Geometry check sheet. Reference: the model listing, model coordinates, mm. Give positions to 0.01 mm unless a question says otherwise; leave off trailing zeros. Order: outer loops, then holes, each group sorted by start corner. A loop starts at its lowest first (then second) coordinate and runs counter-clockwise, first axis right, second up. Notation, with made-up numbers: M 21,18 L 39,18 A10 ccw 39,27 Z; hole C 5,64 d2. An arc over 180 degrees is marked long. Answer as CSV lines item,"result". Start each with the question number.
Q1. Go/stop test with flat-tipped pins: pin 1 (2 mm diameter, centred on x = 30, y = 1.5, fed in from -Z); pin 2 (1 mm diameter, centred on y = 1, z = 15, fed in from -X); pin 3 (0.8 mm diameter, centred on x = -2, y = -1.5, fed in from +Z). Record where each tip stops, or that it passes through.
Q2. Thickness scan on line 1 (X direction, y = -1.5, z = 22); line 2 (Z direction, x = -13, y = 0.25). Record the ranges inside material, lowest first.
Q3. Section check A-A, the plane y = -1.1. Record the boundary of the cut face in (x, z).
```python
from build123d import *

# Parameters (mm, degrees)
BOSS_EXTRUDE1_DEPTH = 2.54
BOSS_EXTRUDE2_DEPTH = 2.54
FILLET1_R           = 2.54


with BuildPart() as part:
    # Sketch1 → Boss-Extrude1 (new body)
    with BuildSketch(Plane(origin=(0, 0, 0), x_dir=(1, 0, 0), z_dir=(0, 1, 0))):
        with BuildLine():
            Line((-44.45, 50.8), (44.45, 50.8))
            ThreePointArc((44.45, 50.8), (48.940128061, 48.940128061), (50.8, 44.45))
            Line((50.8, 44.45), (50.8, -44.45))
            ThreePointArc((50.8, -44.45), (48.940128061, -48.940128061), (44.45, -50.8))
            Line((44.45, -50.8), (-44.45, -50.8))
            ThreePointArc((-44.45, -50.8), (-48.940128061, -48.940128061), (-50.8, -44.45))
            Line((-50.8, -44.45), (-50.8, 44.45))
            ThreePointArc((-50.8, 44.45), (-48.940128061, 48.940128061), (-44.45, 50.8))
        make_face()
    extrude(amount=BOSS_EXTRUDE1_DEPTH)

    # Sketch2 → Boss-Extrude2 (add)
    with BuildSketch(Plane.XZ):
        with BuildLine():
            Line((-48.26, 44.45), (-48.26, -44.45))
            ThreePointArc((-48.26, -44.45), (-47.144076836, -47.144076836), (-44.45, -48.26))
            Line((-44.45, -48.26), (44.45, -48.26))
            ThreePointArc((44.45, -48.26), (47.144076836, -47.144076836), (48.26, -44.45))
            Line((48.26, -44.45), (48.26, 44.45))
            ThreePointArc((48.26, 44.45), (47.144076836, 47.144076836), (44.45, 48.26))
            Line((44.45, 48.26), (-44.45, 48.26))
            ThreePointArc((-44.45, 48.26), (-47.144076836, 47.144076836), (-48.26, 44.45))
        make_face()
    extrude(amount=BOSS_EXTRUDE2_DEPTH)

    # Fillet1
    fillet1_edges = [part.edges().sort_by_distance(p)[0] for p in [
        (48.940128061, 2.54, -48.940128061),
        (50.8, 2.54, 0),
        (48.940128061, 2.54, 48.940128061),
        (0, 2.54, 50.8),
        (-48.940128061, 2.54, 48.940128061),
        (-50.8, 2.54, 0),
        (-48.940128061, 2.54, -48.940128061),
        (0, 2.54, -50.8),
    ]]
    fillet(fillet1_edges, radius=FILLET1_R - 0.0001)  # a hair under: the kernel refuses the full size


solid = part.part
```
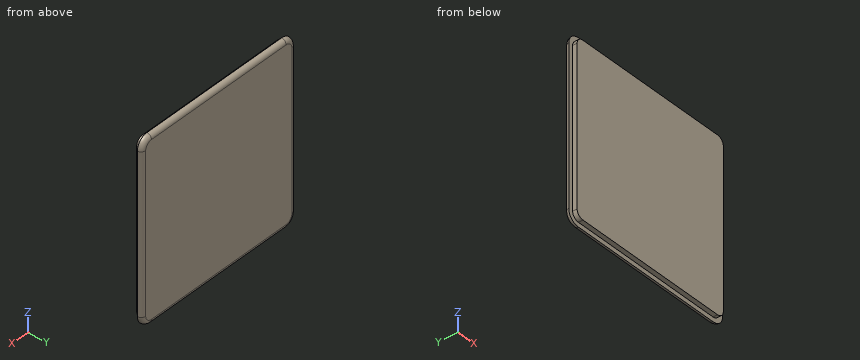
Answer block:
1,pin 1,"stops at z = -50.75"
1,pin 2,"stops at x = -50.75"
1,pin 3,"stops at z = 48.26"
2,line 1,"x = -48.26 to 48.26"
2,line 2,"z = -50.79 to 50.79"
3,outline,"M -48.26,-44.45 A3.81 ccw -44.45,-48.26 L 44.45,-48.26 A3.81 ccw 48.26,-44.45 L 48.26,44.45 A3.81 ccw 44.45,48.26 L -44.45,48.26 A3.81 ccw -48.26,44.45 Z"
